```python
from build123d import *

# Parameters (mm, degrees)
F1_DEPTH = 57.15
F3_DEPTH = 44.45
F4_DEPTH = 44.45
F2_R     = 12.7
F5_DEPTH = 57.151
F6_R     = 5.08
F7_DEPTH = 85.091


with BuildPart() as f1:
    # F0 (on Front) → F1 (new body)
    with BuildSketch(Plane.XZ):
        Polygon((12.7, 0), (63.5, 0), (63.5, 63.5), (-63.5, 63.5), (-63.5, 0), (-12.7, 0), (-12.7, -8.89), (-31.75, -8.89), (-31.75, -21.59), (31.75, -21.59), (31.75, -8.89), (12.7, -8.89), align=None)
    extrude(amount=-F1_DEPTH)

    # F2 (on face) → F3 (cut)
    with BuildSketch(Plane.XZ):
        with BuildLine():
            Line((63.5, 63.5), (0, 63.5))
            ThreePointArc((0, 63.5), (11.952941, 60.511765), (21.093426, 52.250173))
            Line((21.093426, 52.250173), (47.625, 12.7))
            Line((47.625, 12.7), (63.5, 12.7))
            Line((63.5, 12.7), (63.5, 63.5))
        make_face()
    extrude(amount=-F3_DEPTH, mode=Mode.SUBTRACT)

    # F2 (on face) → F4 (cut)
    with BuildSketch(Plane.XZ):
        with BuildLine():
            Line((-47.625, 12.7), (-21.093426, 52.250173))
            ThreePointArc((-21.093426, 52.250173), (-11.952941, 60.511765), (0, 63.5))
            Line((0, 63.5), (-63.5, 63.5))
            Line((-63.5, 63.5), (-63.5, 12.7))
            Line((-63.5, 12.7), (-47.625, 12.7))
        make_face()
    extrude(amount=-F4_DEPTH, mode=Mode.SUBTRACT)

    # F2 (on face) → F5 (cut, through all)
    with BuildSketch(Plane.XZ):
        with Locations((0, 38.1)):
            Circle(F2_R)
    extrude(amount=-F5_DEPTH, mode=Mode.SUBTRACT)

    # F6 (on face) → F7 (cut, through all)
    with BuildSketch(Plane.XY.offset(63.5)):
        with Locations((0, 22.225)):
            Circle(F6_R)
    extrude(amount=-F7_DEPTH, mode=Mode.SUBTRACT)


solid = f1.part
```
Geometry check sheet. Reference: the model listing, model coordinates, mm. A direction names the side the tool comes from. Coordinates: 2 decimals unless noted, no trailing zeros. Order: outer loops, then holes, each group sorted by start corner. A loop starts at its lowest first (then second) coordinate and runs counter-clockwise, first axis right, second up.
Item 1: Scan lines: line 1 along X through (y, z) = (50.5, 38.5); line 2 along Z through (x, y) = (0, 32); line 3 along Y through (x, z) = (0, 16) (3 decimals). Record each from-to range of solid material in increasing order.
Item 2: Mould release check, pull along Z, two halves, no side actions. Record for faces 5 (the flat face through (-1, 57.15, 22)), 6 (the flat face through (34.173, 21.914, 32.752)), 7 (the cylindrical face through (12.114, 28.175, 41.915)), 8 (the flat face through (22, 28, -8.89)): released by +Z, released by -Z, zero draft, split by the parting line, or undercut.
Item 3: Section check B-B (x = -7.5). Enter the section's corners in (y, z), plus the area to 3 significant figures.
Item 4: Section check C-C (y = 47.5). Enter the section's corners in (x, z).
Item 5: Tool access check on faces 1 (the flat face through (-56, 22, 12.7)), 2 (the flat face through (55, 22, 12.7)), 3 (the flat face through (31.75, 28, -15)), 4 (the flat face through (-12.7, 28, -4)). Record the directions out of +Z, -Z, +X, -X, +Y, -Y that give a thin tool (end or side, any length) a straight path to the whole face; none if there is none.
Item 6: Section check D-D (x = 55). Enter the section's corners in (y, z).
Item 7: Depth check by flat-ended pin: pin 1 (4 mm diameter, centred on x = -33.5, y = 18, fed in from +Z); pin 2 (3 mm diameter, centred on x = 39, y = 11.5, fed in from -Z); pin 3 (6 mm diameter, centred on x = 50.5, z = 29, fed in from -Y). Enter the tip coordinate at first touch or a pass-through.
Item 8: Section check A-A (z = 38.1). Enter the section's corners in (x, y), plus the area to 3 significant figures.
Check sheet entries:
1. line 1: x = -63.5 to -12.69, 12.69 to 63.5
1. line 2: z = -21.59 to 25.4, 50.8 to 63.5
1. line 3: y = 0 to 17.145, 27.305 to 57.15
2. face 5: zero draft
2. face 6: released by +Z
2. face 7: undercut
2. face 8: undercut
3. outline: (0, -21.59) - (57.15, -21.59) - (57.15, 27.85) - (0, 27.85) - close; (0, 48.35) - (57.15, 48.35) - (57.15, 63.5) - (44.45, 63.5) - (44.45, 62.37) - (0, 62.37) - close
3. area: 3,640 mm2
4. outline: (-63.5, 0) - (-12.7, 0) - (-12.7, -8.89) - (-31.75, -8.89) - (-31.75, -21.59) - (31.75, -21.59) - (31.75, -8.89) - (12.7, -8.89) - (12.7, 0) - (63.5, 0) - (63.5, 63.5) - (-63.5, 63.5) - close; hole circle Ø25.4 at (0, 38.1)
5. face 1: +Z, -X, -Y
5. face 2: +Z, +X, -Y
5. face 3: -Z, +X, +Y, -Y
5. face 4: -X, +Y, -Y
6. outline: (0, 0) - (57.15, 0) - (57.15, 63.5) - (44.45, 63.5) - (44.45, 12.7) - (0, 12.7) - close
7. pin 1: stops at z = 36.74
7. pin 2: stops at z = 0
7. pin 3: stops at y = 44.45
8. outline: (-63.5, 44.45) - (-30.59, 44.45) - (-30.59, 0) - (-12.7, 0) - (-12.7, 57.15) - (-63.5, 57.15) - close; (12.7, 0) - (30.59, 0) - (30.59, 44.45) - (63.5, 44.45) - (63.5, 57.15) - (12.7, 57.15) - close
8. area: 2,880 mm2
